Verification items for the finished model (mm, model axes). Coordinates: 2 decimals unless noted, no trailing zeros. Write each loop counter-clockwise with the first axis right and the second up, starting at its lowest first coordinate (ties: lowest second). Pieces come first, ordered by that corner, then holes. Notation, with made-up numbers: (49, -24.75) -> (99, -24.75) arc R28 ccw to (99, 12.25) -> close; hole circle Ø6 at (53.5, 66). An arc over 180 degrees is marked (long way). Answer in a Markdown table with one row per item.
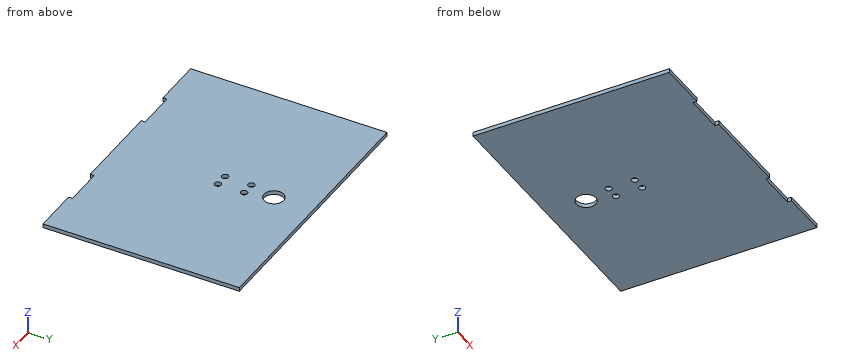
```python
from build123d import *

# Parameters (mm, degrees)
SKETCH1_W           = 203
SKETCH1_H           = 150
BOSS_EXTRUDE1_DEPTH = 3
SKETCH3_R           = 7.5
SKETCH3_R_2         = 2.5
CUT_EXTRUDE2_DEPTH  = 10
SKETCH4_W           = 30
SKETCH4_H           = 3
CUT_EXTRUDE3_DEPTH  = 10


with BuildPart() as part:
    # Sketch1 → Boss-Extrude1 (new body)
    with BuildSketch(Plane.XY):
        Rectangle(SKETCH1_W, SKETCH1_H)
    extrude(amount=BOSS_EXTRUDE1_DEPTH)

    # Sketch3 → Cut-Extrude2 (cut)
    with BuildSketch(Plane.XY.offset(3)):
        with Locations((0, 45)):
            Circle(SKETCH3_R)
        with Locations((-5, 25)):
            Circle(SKETCH3_R_2)
        with Locations((-5, 5)):
            Circle(SKETCH3_R_2)
        with Locations((5, 5)):
            Circle(SKETCH3_R_2)
        with Locations((5, 25)):
            Circle(SKETCH3_R_2)
    extrude(amount=-CUT_EXTRUDE2_DEPTH, mode=Mode.SUBTRACT)

    # Sketch4 → Cut-Extrude3 (cut)
    with BuildSketch(Plane.XY.offset(3)):
        with Locations((-48.5, -73.5)):
            Rectangle(SKETCH4_W, SKETCH4_H)
        with Locations((51.5, -73.5)):
            Rectangle(SKETCH4_W, SKETCH4_H)
    extrude(amount=-CUT_EXTRUDE3_DEPTH, mode=Mode.SUBTRACT)


solid = part.part
```
1. Section check A-A, the plane y = 25. Record the boundary of the cut face in (x, z), plus the area to 3 significant figures.
Geometry says:
| item | result |
|---|---|
| outline | (-101.5, 0) -> (-7.5, 0) -> (-7.5, 3) -> (-101.5, 3) -> close; (-2.5, 0) -> (2.5, 0) -> (2.5, 3) -> (-2.5, 3) -> close; (7.5, 0) -> (101.5, 0) -> (101.5, 3) -> (7.5, 3) -> close |
| area | 579 mm^2 |
2. Depth check by flat-ended pin: P1, Ø19.5, axis at x = 0, y = 45, coming from the +Z side. Enter the tip coordinate at first touch or a pass-through.
Geometry says:
| item | result |
|---|---|
| P1 | z = 3 |
3. Thickness scan on line 1 (Y direction, x = 0, z = 1.25); line 2 (Y direction, x = 5, z = 1.8); line 3 (Y direction, x = 4.5, z = 0.7). Record the ranges inside material, lowest first. Write a range as from..to.
Geometry says:
| item | result |
|---|---|
| line 1 | -75..37.5, 52.5..75 |
| line 2 | -75..2.5, 7.5..22.5, 27.5..39.41, 50.59..75 |
| line 3 | -75..2.55, 7.45..22.55, 27.45..39, 51..75 |
4. Section check B-B, the plane x = -5. Record the boundary of the cut face in (y, z).
Geometry says:
| item | result |
|---|---|
| outline | (-75, 0) -> (2.5, 0) -> (2.5, 3) -> (-75, 3) -> close; (7.5, 0) -> (22.5, 0) -> (22.5, 3) -> (7.5, 3) -> close; (27.5, 0) -> (39.41, 0) -> (39.41, 3) -> (27.5, 3) -> close; (50.59, 0) -> (75, 0) -> (75, 3) -> (50.59, 3) -> close |
5. Section check D-D, the plane x = 46. Record the boundary of the cut face in (y, z), plus the area to 3 significant figures.
Geometry says:
| item | result |
|---|---|
| outline | (-72, 0) -> (75, 0) -> (75, 3) -> (-72, 3) -> close |
| area | 441 mm^2 |
6. Section check C-C, the plane y = 45. Record the boundary of the cut face in (x, z).
Geometry says:
| item | result |
|---|---|
| outline | (-101.5, 0) -> (-7.5, 0) -> (-7.5, 3) -> (-101.5, 3) -> close; (7.5, 0) -> (101.5, 0) -> (101.5, 3) -> (7.5, 3) -> close |
